Autodesk Fusion 360 part; units mm, degrees
sketch "Wheel_Ax_Sketch" plane through (0, 0, 0) normal (0, 0, 1) x (1, 0, 0)
  arc A0 (-3, 3) -> (-3, -3) centre (0, 0) ccw
  arc A1 (-3, 3) -> (-3, -3) centre (0, 0) ccw
  line L0 (-3, -3) -> (3, -3)
  arc A2 (3, -3) -> (3, 3) centre (0, 0) ccw
  line L1 (3, 3) -> (-3, 3)
  circle A3 centre (0, 0) radius 5
  dimension "d1" = 10
extrude "Extrude1" add sketch "Wheel_Ax_Sketch" along normal blind 47.5 contours A0 A1 L0 A2 L1
extrude "Extrude2" add sketch "Wheel_Ax_Sketch" along normal blind 2.2 from surface at 9.5
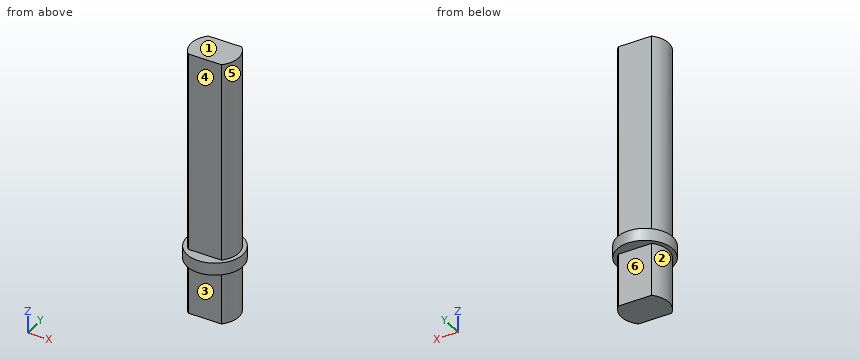
Design review of the part built by this model. Coordinates are the model's own, in mm. Face numbers are marked on the shaded views. A direction names the side the tool comes from. Coordinates: 2 decimals unless noted, no trailing zeros. Write each loop counter-clockwise with the first axis right and the second up, starting at its lowest first coordinate (ties: lowest second). Pieces come first, ordered by that corner, then holes. Notation, with made-up numbers: (37, 63.25) - (77, 63.25) arc R24 cw to (77, 83.25) - close; hole circle Ø7 at (-16, 26). An arc over 180 degrees is marked (long way). One line per item, written item: value.
1) Add section C-C (z = 8.5). State the section outline as (x, y) points.
Answer sheet:
outline: (-3, -3) - (3, -3) arc R4.24 ccw to (3, 3) - (-3, 3) arc R4.24 ccw to start
2) Add section D-D (y = 3.5). State the section outline as (x, z) points.
Answer sheet:
outline: (-3.57, 9.5) - (3.57, 9.5) - (3.57, 11.7) - (-3.57, 11.7) - close
3) To check wall thickness, follow probe 1 along X at (y, z) = (0, 22); probe 2 along Y at (x, z) = (-2.5, 41.5); probe 3 along Z at (x, y) = (1.5, -3.25). State the ranges of each line that lie inside material, in increasing order.
Answer sheet:
probe 1: x = -4.24 to 4.24
probe 2: y = -3 to 3
probe 3: z = 9.5 to 11.7
4) Insertion check: pin 1 (4 mm diameter, centred on x = 1, y = 2.5, fed in from -Z); pin 2 (4 mm diameter, centred on x = 1.5, z = 27, fed in from +Y); pin 3 (4 mm diameter, centred on y = -3, z = 6, fed in from +X); pin 4 (5 mm diameter, centred on x = 0.5, z = 24.5, fed in from -Y). Each pin has a flat end and moves straight along its axis. Give the tip position at first contact, or say it passes through.
Answer sheet:
pin 1: stops at z = 0
pin 2: stops at y = 3
pin 3: stops at x = 4.12
pin 4: stops at y = -3
5) Add section B-B (y = 0). State the section outline as (x, z) points.
Answer sheet:
outline: (-5, 9.5) - (-4.24, 9.5) - (-4.24, 0) - (4.24, 0) - (4.24, 9.5) - (5, 9.5) - (5, 11.7) - (4.24, 11.7) - (4.24, 47.5) - (-4.24, 47.5) - (-4.24, 11.7) - (-5, 11.7) - close
6) Add section A-A (x = 0). State the section outline as (y, z) points.
Answer sheet:
outline: (-5, 9.5) - (-3, 9.5) - (-3, 0) - (3, 0) - (3, 9.5) - (5, 9.5) - (5, 11.7) - (3, 11.7) - (3, 47.5) - (-3, 47.5) - (-3, 11.7) - (-5, 11.7) - close
7) Mouldability with a two-part tool opening along Y and no side actions: class the marked faces 1, 2 and 3 as +Y half, -Y half, draft (parallel to the pull), parting line (faces both ways), or undercut.
Answer sheet:
face 1: draft
face 2: parting line
face 3: -Y half
8) For the marked faces 4, 5 and 6, list the 3-axis set-ups (+Z, -Z, +X, -X, +Y, -Y) from which the entire face can be reached by the end or side of a thin tool; tool diameter is ignored.
Answer sheet:
face 4: +Z, +X, -X, -Y
face 5: +Z, +X
face 6: -Z, +X, -X, +Y
